Source: CAD feature listing. Evaluate the final solid. Frame: model axes, mm. Face numbers are marked on the shaded views. A direction names the side the tool comes from. Coordinates: 2 decimals unless noted, no trailing zeros. Write each loop counter-clockwise with the first axis right and the second up, starting at its lowest first coordinate (ties: lowest second). Pieces come first, ordered by that corner, then holes. Notation, with made-up numbers: M 61.5,20.5 L 115.5,20.5 A19 ccw 115.5,27.5 Z; hole C -0.75,84 d8. An arc over 180 degrees is marked long. One line per item, written item: value. Start each with the question number.
Item 1: Set-up query: the marked faces 4, 5, 6 and 7. Return all of +Z, -Z, +X, -X, +Y, -Y with unobstructed straight access to the full face (end or side cutting, diameter ignored); none if empty.
Item 2: Cut plane C-C, the plane z = -170. Output: boundary loops of the cut face in (x, y).
Item 3: Cut plane A-A, the plane z = -69. Output: boundary loops of the cut face in (x, y), then the cut area to 3 significant figures.
Item 4: Cut plane D-D, the plane y = -2. Output: boundary loops of the cut face in (x, z).
Item 5: Ray query, L1, parallel to Y at x = 16.5, z = -94.5; L2, parallel to Y at x = 1, z = -170; L3, parallel to Z at x = 0, y = 54.25. Return the intervals inside material, ascending. Write a range as from..to.
Item 6: Mould query, pull axis Y, two halves, no side actions, for the marked faces 1, 2 and 3. Classes: released by +Y, released by -Y, zero draft, split by the parting line, or undercut.
Item 7: Cut plane B-B, the plane x = 12. Output: boundary loops of the cut face in (y, z).
Item 8: Pin query (flat end, axial travel): P1, Ø18, axis at x = 0, z = 0, coming from the +Y side; P2, Ø20, axis at x = 7, y = 30.5, coming from the +Z side; P3, Ø3, axis at x = 3.5, z = -114.5, coming from the -Y side; P4, Ø1, axis at x = -7, y = 57.5, coming from the +Z side. Return the tip coordinate at first contact, or that it passes through.
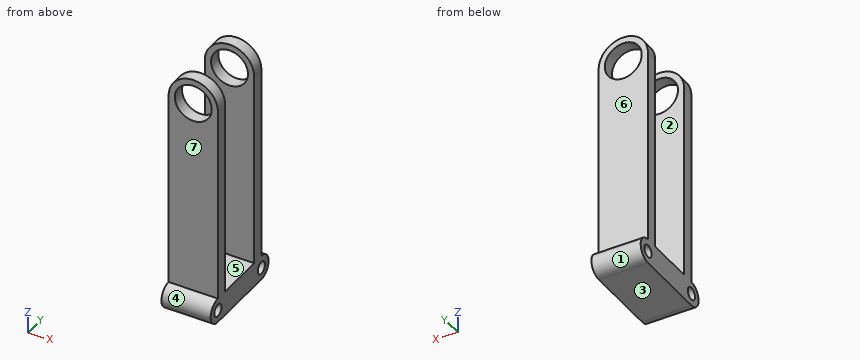
```python
from build123d import *

# Parameters (mm, degrees)
SKETCH_1_R           = 15
EXTRUDE_1_DEPTH      = 60
SKETCH_2_W           = 40
SKETCH_2_H           = 40
CUT_EXTRUDE_1_DEPTH  = 190
EXTRUDE_2_DEPTH      = 50
EXTRUDE_2_DEPTH_BACK = 10
SKETCH_4_R           = 10
EXTRUDE_3_DEPTH      = 40
SKETCH_5_R           = 5
CUT_EXTRUDE_3_DEPTH  = 40


with BuildPart() as part:
    # Sketch 1 → Extrude 1 (new body)
    with BuildSketch(Plane(origin=(0, 0, 0), x_dir=(1, 0, 0), z_dir=(0, 1, 0))):
        with BuildLine():
            Line((20, 0), (20, 170))
            Line((20, 170), (-20, 170))
            Line((-20, 170), (-20, 0))
            ThreePointArc((-20, 0), (0, -20), (20, 0))
        make_face()
        with Locations(Location((0, 0, 0), (0, 0, 270))):
            Circle(SKETCH_1_R, mode=Mode.SUBTRACT)
    extrude(amount=EXTRUDE_1_DEPTH)

    # Sketch 2 → Cut-Extrude 1 (cut)
    with BuildSketch(Plane(origin=(0, 0, -170), x_dir=(-1, 0, 0), z_dir=(0, 0, -1))):
        with Locations((0, 30)):
            Rectangle(SKETCH_2_W, SKETCH_2_H)
    extrude(amount=-CUT_EXTRUDE_1_DEPTH, mode=Mode.SUBTRACT)


with BuildPart() as cut_extrude_1_piece_1:
    # of the separate pieces the step leaves, piece 1, a body of its own (cut_extrude_1_pieces)
    add(part.part.solids().sort_by_distance((20, 50, -170))[0])



with BuildPart() as cut_extrude_1_piece_2:
    # of the separate pieces the step leaves, piece 2, a body of its own (cut_extrude_1_pieces)
    add(part.part.solids().sort_by_distance((20, 0, 0))[0])


with BuildPart() as cut_extrude_1_piece_1_1:
    add(cut_extrude_1_piece_1.part)

    add(cut_extrude_1_piece_2.part)  # Extrude 2 merges Cut-Extrude 1 piece 2
    # Sketch 3 → Extrude 2 (add, two sides: drawn at the far end of the back side and taken through both)
    with BuildSketch(Plane(origin=(0, 10, 0), x_dir=(1, 0, 0), z_dir=(0, 1, 0)).offset(-EXTRUDE_2_DEPTH_BACK)):
        Polygon((20, 170), (20, 160), (-20, 160), (-20, 170), (-20, 180), (20, 180), align=None)
    extrude(amount=EXTRUDE_2_DEPTH + EXTRUDE_2_DEPTH_BACK)

    # Sketch 4 → Extrude 3 (add)
    with BuildSketch(Plane.ZY.offset(20)):
        with Locations((-170, 0)):
            Circle(SKETCH_4_R)
        with Locations((-170, 60)):
            Circle(SKETCH_4_R)
    extrude(amount=-EXTRUDE_3_DEPTH)

    # Sketch 5 → Cut-Extrude 3 (cut)
    with BuildSketch(Plane.ZY.offset(20)):
        with Locations((-170, 0)):
            Circle(SKETCH_5_R)
        with Locations((-170, 60)):
            Circle(SKETCH_5_R)
    extrude(amount=-CUT_EXTRUDE_3_DEPTH, mode=Mode.SUBTRACT)


solid = cut_extrude_1_piece_1_1.part
```
From the geometry:
1. face 4: +X, -X, -Y
1. face 5: +Z, +X, -X
1. face 6: +Z, +X, -X, +Y
1. face 7: +Z, +X, -X, -Y
2. outline: M -20,-10 L 20,-10 L 20,-5 L -20,-5 Z; M -20,5 L 20,5 L 20,55 L -20,55 Z; M -20,65 L 20,65 L 20,70 L -20,70 Z
3. outline: M -20,0 L 20,0 L 20,10 L -20,10 Z; M -20,50 L 20,50 L 20,60 L -20,60 Z
3. area: 800 mm²
4. outline: M -20,-179.8 L 20,-179.8 L 20,-174.58 L -20,-174.58 Z; M -20,-165.42 L 20,-165.42 L 20,-160.2 L -20,-160.2 Z
5. L1: y = 0..10, 50..60
5. L2: y = -10..-5, 5..55, 65..70
5. L3: z = -180..-15, 15..20
6. face 1: released by +Y
6. face 2: undercut
6. face 3: zero draft
7. outline: M 0,-180 L 60,-180 A10 ccw 60,-160 L 60,-9 L 50,-9 L 50,-160 L 10,-160 L 10,-9 L 0,-9 L 0,-160 A10 ccw Z; M 0,9 L 10,9 L 10,16 L 0,16 Z; M 50,9 L 60,9 L 60,16 L 50,16 Z; hole C 0,-170 d10; hole C 60,-170 d10
8. P1: passes through
8. P2: stops at z = -160
8. P3: stops at y = 0
8. P4: stops at z = 18.91
